from build123d import *

# Parameters (mm, degrees)
F1_DEPTH = 20


with BuildPart() as f1:
    # F0 (on Front) → F1 (new body)
    with BuildSketch(Plane.XZ):
        with BuildLine():
            ThreePointArc((-49.7328845509, 82.027652927), (-54.3163875498, 81.6524498366), (-58.8995327156, 81.2729007771))
            ThreePointArc((-58.8995327156, 81.2729007771), (-129.6276844332, 1.8675286407), (-62.5862937495, -80.6741971997))
            ThreePointArc((-62.5862937495, -80.6741971997), (-54.3983095736, -81.3659722205), (-46.209165104, -82.0438736892))
            ThreePointArc((-46.209165104, -82.0438736892), (10.915997147, -57.5305572299), (34.4621609717, 0))
            ThreePointArc((34.4621609717, 0), (9.6672248523, 58.7735942734), (-49.7328845509, 82.027652927))
        make_face()
        with BuildLine():
            ThreePointArc((738.1113483102, 81.9430534241), (344.1909525373, 98.009208707), (-49.7328845509, 82.027652927))
            ThreePointArc((-49.7328845509, 82.027652927), (9.6672248523, 58.7735942734), (34.4621609717, 0))
            Line((34.4621609717, 0), (660.3510609717, 0))
            ThreePointArc((660.3510609717, 0), (682.8853398752, 56.4830202172), (738.1113483102, 81.9430534241))
        make_face()
        with BuildLine():
            ThreePointArc((34.4621609717, 0), (10.915997147, -57.5305572299), (-46.209165104, -82.0438736892))
            ThreePointArc((-46.209165104, -82.0438736892), (350.9486567166, -98.2391856001), (748.0988502502, -81.8578749895))
            ThreePointArc((748.0988502502, -81.8578749895), (686.433253644, -60.0008046218), (660.3510609717, 0))
            Line((660.3510609717, 0), (34.4621609717, 0))
        make_face()
        with BuildLine():
            ThreePointArc((824.4621609717, 0), (798.8896311889, 59.5212710965), (738.1113483102, 81.9430534241))
            ThreePointArc((738.1113483102, 81.9430534241), (682.8853398752, 56.4830202172), (660.3510609717, 0))
            ThreePointArc((660.3510609717, 0), (686.433253644, -60.0008046218), (748.0988502502, -81.8578749895))
            ThreePointArc((748.0988502502, -81.8578749895), (802.4074155935, -55.9733573277), (824.4621609717, 0))
        make_face()
    extrude(amount=F1_DEPTH)


solid = f1.part
Could you check a few things on this model? Use its own coordinates, in mm. Give positions to 0.01 mm unless a question says otherwise; leave off trailing zeros. Loops run counter-clockwise (first coordinate to the right, second up) from the corner with the lowest first, then second, coordinate; pieces in that order, holes last. Notation, with made-up numbers: (56, 87) -> (71, 87) arc R26 ccw to (71, 124) -> close; hole circle Ø7 at (26.5, 36). An arc over 180 degrees is marked (long way). Answer as CSV lines item,"result". Start each with the question number.
(1) I need wall thicknesses on probe 1 along X at (y, z) = (-5, 1.5); probe 2 along Z at (x, y) = (363, -15); probe 3 along X at (y, z) = (-16.5, 1). Which ranges of each line are inside material? Lowest first, please.
(2) If we section it at A-A on y = -16: Write out the boundary of the cut face in (x, z), then the cut area to 3 significant figures.
(3) If we section it at C-C on z = -68: Write out the boundary of the cut face in (x, y).
(4) I'm going to push flat-ended pins straight in: pin 1 Ø5 at (y, z) = (-17, 62.5) entering from -X; pin 2 Ø1 at (x, z) = (314, 69.5) entering from +Y; pin 3 Ø12 at (y, z) = (-12.5, 62.5) entering from -X; pin 4 Ø12 at (y, z) = (-14.5, 60) entering from +X. Where does each tip first touch, or does it pass through?
(5) If we section it at B-B on x = 542: Write out the boundary of the cut face in (y, z).
Computed:
1,probe 1,"x = -129.64 to 824.45"
1,probe 2,"z = -98.22 to 97.97"
1,probe 3,"x = -129.64 to 824.46"
2,outline,"(-62.59, -80.67) arc R4850 ccw to (-46.21, -82.04) arc R4850 ccw to (748.1, -81.86) arc R82.06 ccw to (738.11, 81.94) arc R4850 ccw to (-49.73, 82.03) arc R4850 ccw to (-58.9, 81.27) arc R82.06 ccw to start"
2,area,"168,000 mm2"
3,outline,"(-93.52, -20) -> (788.33, -20) -> (788.33, 0) -> (-93.52, 0) -> close"
4,pin 1,"stops at x = -103.57"
4,pin 2,"stops at y = 0"
4,pin 3,"stops at x = -107.1"
4,pin 4,"stops at x = 804.19"
5,outline,"(-20, -94.43) -> (0, -94.43) -> (0, 93.95) -> (-20, 93.95) -> close"
